from build123d import *

# Parameters (mm, degrees)
F0_W     = 40
F0_H     = 22
F1_DEPTH = 2
F2_W     = 22
F2_H     = 22
F3_DEPTH = 25
F4_R     = 3


with BuildPart() as f1:
    # F0 (on Top) → F1 (new body)
    with BuildSketch(Plane.XY):
        with Locations((-4.791172, 0.456456)):
            Rectangle(F0_W, F0_H)
    extrude(amount=F1_DEPTH)

    # F2 (on face) → F3 (join)
    with BuildSketch(Plane.XY.offset(2)):
        with Locations((4.208828, 0.456456)):
            Rectangle(F2_W, F2_H)
    extrude(amount=F3_DEPTH)

    # F4
    f4_edges = [f1.edges().sort_by_distance(p)[0] for p in [
        (-24.791172, 11.456456, 1),
        (-24.791172, -10.543544, 1),
        (15.208828, -10.543544, 13.5),
        (15.208828, 0.456456, 0),
        (15.208828, 11.456456, 13.5),
        (15.208828, 0.456456, 27),
    ]]
    fillet(f4_edges, radius=F4_R)


solid = f1.part
Source: CAD feature listing. Evaluate the final solid. Frame: model axes, mm. A direction names the side the tool comes from. Give positions to 0.01 mm unless a question says otherwise; leave off trailing zeros. Write each loop counter-clockwise with the first axis right and the second up, starting at its lowest first coordinate (ties: lowest second). Pieces come first, ordered by that corner, then holes. Notation, with made-up numbers: (81, 58) -> (114, 58) arc R30 cw to (114, 94) -> close; hole circle Ø5 at (13.5, 9.5). An arc over 180 degrees is marked (long way). Return JSON: item names as keys, results as strings. Group by question number.
1. Access query for faces 1 (the face through (-6.791, 0, 14)), 2 (the face through (3, 11.456, 13)). Directions: +Z, -Z, +X, -X, +Y, -Y. A direction counts if a zero-diameter tool reaches every point of the face in a straight line with its end or side. Return the directions, or none.
2. Section A-A, the plane y = -4.5. Output: boundary loops of the cut face in (x, z), then the cut area to 3 significant figures.
3. Section C-C, the plane x = -20.5. Output: boundary loops of the cut face in (y, z).
4. Material intervals for line 1 (Z direction, x = -7, y = -8); line 2 (X direction, y = 0.75, z = 7); line 3 (X direction, y = -8.75, z = 13), sorted ascending. Write a range as from..to.
5. Pin query (flat end, axial travel): pin 1 Ø1.5 at (x, y) = (-12, -7) entering from +Z; pin 2 Ø11 at (y, z) = (-5, 8.5) entering from -X. Return the tip coordinate at first contact, or that it passes through.
6. Section B-B, the plane z = 17. Output: boundary loops of the cut face in (x, y).
Determined:
{
 "1": {"face 1": "+Z, -X, +Y, -Y", "face 2": "+Z, -Z, +X, -X, +Y"},
 "2": {"outline": "(-24.79, 0) -> (12.21, 0) arc R3 ccw to (15.21, 3) -> (15.21, 24) arc R3 ccw to (12.21, 27) -> (-6.79, 27) -> (-6.79, 2) -> (-24.79, 2) -> close", "area": "626 mm2"},
 "3": {"outline": "(-10.54, 0) -> (11.46, 0) -> (11.46, 2) -> (-10.54, 2) -> close"},
 "4": {"line 1": "z = 0..2", "line 2": "x = -6.79..15.21", "line 3": "x = -6.79..14.96"},
 "5": {"pin 1": "stops at z = 2", "pin 2": "stops at x = -6.79"},
 "6": {"outline": "(-6.79, -10.54) -> (12.21, -10.54) arc R3 ccw to (15.21, -7.54) -> (15.21, 8.46) arc R3 ccw to (12.21, 11.46) -> (-6.79, 11.46) -> close"}
}
